Verification items for this drawing (mm, ordinates from the low corner). Coordinates: 2 decimals unless noted, no trailing zeros. Write each loop counter-clockwise with the first axis right and the second up, starting at its lowest first coordinate (ties: lowest second). Pieces come first, ordered by that corner, then holes. Notation, with made-up numbers: (-14, 83.5) -> (36, 83.5) arc R25 ccw to (36, 96.5) -> close; hole circle Ø6 at (-14, -31). An arc over 180 degrees is marked (long way). One line per question, with ' | ' between items.
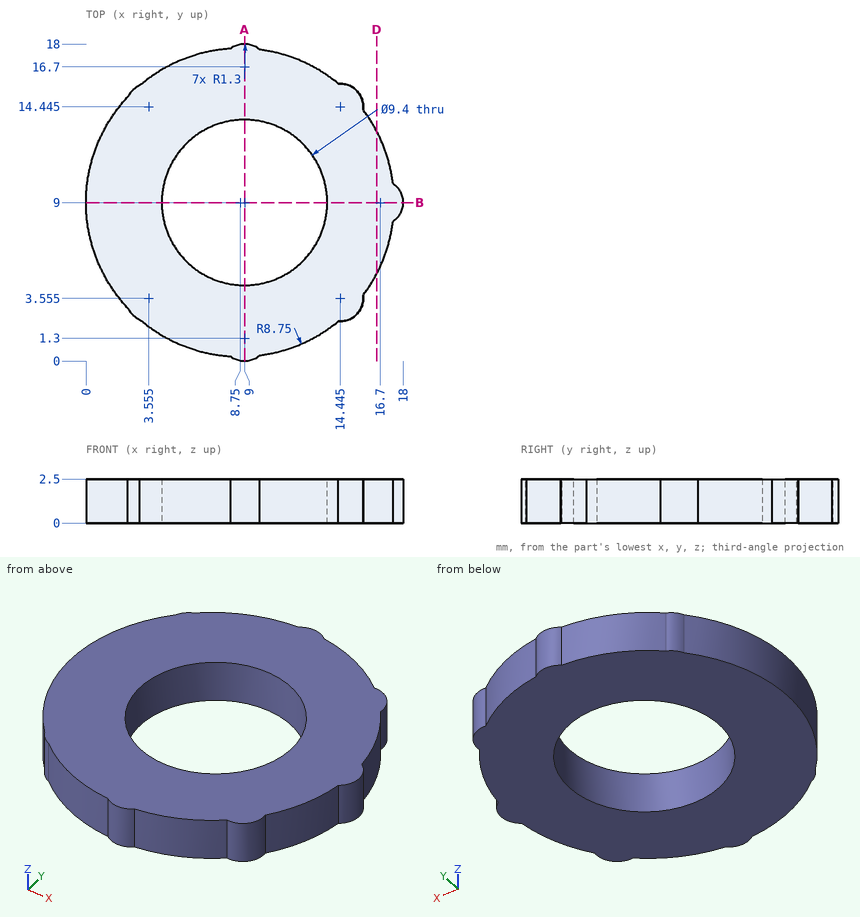
(1) Depth check by flat-ended pin: P1, Ø1, axis at x = 7.5, z = 1, coming from the +Y side. Enter the tip coordinate at first touch or a pass-through.
Answers below:
P1: stops at y = 17.72
(2) Material ranges on line 1 (Y direction, x = 9, z = 1.15); line 2 (X direction, y = 4.75, z = 1.85) (1 decimal); line 3 (Y direction, x = 6, z = 0.25), recorded low to high.
Answers below:
line 1: y = 0 to 4.3, 13.7 to 18 | line 2: x = 1.1 to 7, 11 to 16.4 | line 3: y = 0.69 to 5.38, 12.62 to 17.31
(3) Cross-section at D-D (x = 16.5). Record the cut outline in (y, z).
Answers below:
outline: (4.94, 0) -> (13.06, 0) -> (13.06, 2.5) -> (4.94, 2.5) -> close
(4) Cross-section at A-A (x = 9). Record the cut outline in (y, z).
Answers below:
outline: (0, 0) -> (4.3, 0) -> (4.3, 2.5) -> (0, 2.5) -> close; (13.7, 0) -> (18, 0) -> (18, 2.5) -> (13.7, 2.5) -> close
